The model under review builds one solid part; all positions refer to its coordinate system, in mm. A direction names the side the tool comes from. Coordinates: 2 decimals unless noted, no trailing zeros. Write each loop counter-clockwise with the first axis right and the second up, starting at its lowest first coordinate (ties: lowest second). Pieces come first, ordered by that corner, then holes. Notation, with made-up numbers: (9.5, 23.25) - (32.5, 23.25) arc R16 ccw to (32.5, 31.25) - close; hole circle Ø6 at (52, 57.25). An arc over 180 degrees is marked (long way). Put each result on its own line as item: value.
from build123d import *

# Parameters (mm, degrees)
SKETCH_1_W          = 87.5
SKETCH_1_H          = 28
EXTRUDE_1_DEPTH     = 3
SKETCH_2_R          = 1.25
SKETCH_2_W          = 77.5
SKETCH_2_H          = 22.5
CUT_EXTRUDE_1_DEPTH = 44
CHAMFER_1_SIZE      = 1
SKETCH_4_W          = 1.8
SKETCH_4_H          = 10
CUT_EXTRUDE_2_DEPTH = 92
SKETCH_5_W          = 3
SKETCH_5_H          = 3
EXTRUDE_2_DEPTH     = 87.5
EXTRUDE_3_DEPTH     = 3
SKETCH_8_W          = 77.5
SKETCH_8_H          = 3
CUT_EXTRUDE_3_DEPTH = 4
CHAMFER_3_SIZE      = 2
SKETCH_9_W          = 77.5
SKETCH_9_H          = 3
EXTRUDE_4_DEPTH     = 3
SKETCH_10_W         = 87.5
SKETCH_10_H         = 3
CUT_EXTRUDE_4_DEPTH = 3
CHAMFER_4_SIZE      = 3


with BuildPart() as part:
    # 草图1 → 凸台-拉伸1 (new body)
    with BuildSketch(Plane.XY):
        with Locations((0.266227181, -2.000151732)):
            Rectangle(SKETCH_1_W, SKETCH_1_H)
    extrude(amount=EXTRUDE_1_DEPTH)

    # 草图2 → 切除-拉伸1 (cut)
    with BuildSketch(Plane.XY.offset(3)):
        with Locations((-41.233772819, 7.999848268)):
            Circle(SKETCH_2_R)
        with Locations((-41.233772819, -13.000151732)):
            Circle(SKETCH_2_R)
        with Locations((41.766227181, -13.000151732)):
            Circle(SKETCH_2_R)
        with Locations((41.766227181, 7.999848268)):
            Circle(SKETCH_2_R)
        with Locations((0.266227181, 0.749848268)):
            Rectangle(SKETCH_2_W, SKETCH_2_H)
    extrude(amount=-CUT_EXTRUDE_1_DEPTH, mode=Mode.SUBTRACT)

    # 倒角1
    chamfer_1_edges = [part.edges().sort_by_distance(p)[0] for p in [
        (44.016227181, -16.000151732, 1.5),
        (-43.483772819, -16.000151732, 1.5),
    ]]
    chamfer(chamfer_1_edges, length=CHAMFER_1_SIZE)

    # 草图4 → 切除-拉伸2 (cut)
    with BuildSketch(Plane(origin=(44.016227181, 0, 0), x_dir=(0, 0, -1), z_dir=(1, 0, 0))):
        with Locations((-0.9, -1.000151732)):
            Rectangle(SKETCH_4_W, SKETCH_4_H)
    extrude(amount=-CUT_EXTRUDE_2_DEPTH, mode=Mode.SUBTRACT)

    # 草图5 → 凸台-拉伸2 (add)
    with BuildSketch(Plane(origin=(44.016227181, 0, 0), x_dir=(0, 0, -1), z_dir=(1, 0, 0))):
        with Locations((-1.5, 13.499848268)):
            Rectangle(SKETCH_5_W, SKETCH_5_H)
    extrude(amount=-EXTRUDE_2_DEPTH)

    # 草图7 → 凸台-拉伸3 (add)
    with BuildSketch(Plane(origin=(0, 0, 0), x_dir=(-1, 0, 0), z_dir=(0, 0, -1))):
        Polygon((-44.016227181, -15.000151732), (-44.016227181, -18.000151732), (43.483772819, -18.000151732), (43.483772819, -15.000151732), (42.983772819, -15.500151732), (-43.016227181, -16.000151732), align=None)
    extrude(amount=-EXTRUDE_3_DEPTH)

    # 草图8 → 切除-拉伸3 (cut)
    with BuildSketch(Plane(origin=(0, -10.500151732, 0), x_dir=(1, 0, 0), z_dir=(0, 1, 0))):
        with Locations((0.266227181, -1.5)):
            Rectangle(SKETCH_8_W, SKETCH_8_H)
    extrude(amount=-CUT_EXTRUDE_3_DEPTH, mode=Mode.SUBTRACT)

    # 倒角3
    chamfer_3_edges = [part.edges().sort_by_distance(p)[0] for p in [
        (44.016227181, -18.000151732, 1.5),
        (-43.483772819, -18.000151732, 1.5),
    ]]
    chamfer(chamfer_3_edges, length=CHAMFER_3_SIZE)

    # 草图9 → 凸台-拉伸4 (add)
    with BuildSketch(Plane.XZ.offset(-11.999848268)):
        with Locations((0.266227181, 1.5)):
            Rectangle(SKETCH_9_W, SKETCH_9_H)
    extrude(amount=EXTRUDE_4_DEPTH)

    # 草图10 → 切除-拉伸4 (cut)
    with BuildSketch(Plane(origin=(0, 14.999848268, 0), x_dir=(1, 0, 0), z_dir=(0, 1, 0))):
        with Locations((0.266227181, -1.5)):
            Rectangle(SKETCH_10_W, SKETCH_10_H)
    extrude(amount=-CUT_EXTRUDE_4_DEPTH, mode=Mode.SUBTRACT)

    # 倒角4
    chamfer_4_edges = [part.edges().sort_by_distance(p)[0] for p in [
        (-43.483772819, 11.999848268, 1.5),
        (44.016227181, 11.999848268, 1.5),
    ]]
    chamfer(chamfer_4_edges, length=CHAMFER_4_SIZE)


solid = part.part
1. Consider section C-C on z = 0.5. State the section outline as (x, y) points.
Determined:
outline: (-43.48, -16) - (-41.48, -18) - (42.02, -18) - (44.02, -16) - (44.02, -6) - (39.02, -6) - (39.02, -14.5) - (-38.48, -14.5) - (-38.48, -6) - (-43.48, -6) - close; (-43.48, 4) - (-38.48, 4) - (-38.48, 9) - (39.02, 9) - (39.02, 4) - (44.02, 4) - (44.02, 9) - (41.02, 12) - (-40.48, 12) - (-43.48, 9) - close; hole circle Ø2.5 at (-41.23, -13); hole circle Ø2.5 at (-41.23, 8); hole circle Ø2.5 at (41.77, -13); hole circle Ø2.5 at (41.77, 8)
2. Machinability: for faces 5 (the flat face through (-41, -1, 1.8)), 6 (the flat face through (11, -15, 0)), 7 (the flat face through (0, -14.5, 1)), which of the approach directions +Z, -Z, +X, -X, +Y, -Y give a long, thin tool a straight path to every point of the face, cutting with its end or side? Answer none if there is none.
Determined:
face 5: -Z, +X, -X
face 6: -Z, +X, -X, +Y, -Y
face 7: +Z, -Z
3. For pin 1 Ø4 at (x, y) = (42, -1) entering from -Z; pin 2 Ø1.4 at (x, z) = (-42, 1) entering from +Y; pin 3 Ø0.5 at (x, z) = (43, 1) entering from +Y; pin 4 Ø4 at (x, y) = (-41.23, -13) entering from -Z, all flat-tipped, find the tip position at first contact; note any pin that passes through.
Determined:
pin 1: stops at z = 1.8
pin 2: stops at y = 11.18
pin 3: stops at y = 10.27
pin 4: stops at z = 0
4. The part is to be moulded in two halves that separate along Y. For faces 1 (the flat face through (43.002, -17.014, 1.479)), 2 (the flat face through (-6, -15, 3)), 3 (the flat face through (0, 12, 1)), 4 (the flat face through (-38.484, -3, 2)), say which applies: +Y half, -Y half, draft (parallel to the pull), parting line (faces both ways), or undercut.
Determined:
face 1: -Y half
face 2: draft
face 3: +Y half
face 4: undercut
5. Consider section A-A on y = -5. State the section outline as (x, z) points, plus the area to 3 significant figures.
Determined:
outline: (-43.48, 1.8) - (-38.48, 1.8) - (-38.48, 3) - (-43.48, 3) - close; (39.02, 1.8) - (44.02, 1.8) - (44.02, 3) - (39.02, 3) - close
area: 12.0 mm^2
6. Consider section B-B on x = 29.5. State the section outline as (y, z) points, plus the area to 3 significant figures.
Determined:
outline: (-18, 0) - (-14.5, 0) - (-14.5, 3) - (-18, 3) - close; (9, 0) - (12, 0) - (12, 3) - (9, 3) - close
area: 19.5 mm^2
7. To check wall thickness, follow probe 1 along Y at (x, z) = (11, 1.95); probe 2 along X at (y, z) = (6, 1.8); probe 3 along X at (y, z) = (7.25, 2.7). State the ranges of each line that lie inside material, in increasing order.
Determined:
probe 1: y = -18 to -14.5, 9 to 12
probe 2: x = -43.48 to -38.48, 39.02 to 44.02
probe 3: x = -43.48 to -42.23, -40.23 to -38.48, 39.02 to 40.77, 42.77 to 44.02
